Model file for the job. Use its own axes, mm. A direction names the side the tool comes from. Coordinates: 2 decimals unless noted, no trailing zeros. Order: outer loops, then holes, each group sorted by start corner. A loop starts at its lowest first (then second) coordinate and runs counter-clockwise, first axis right, second up. Notation, with made-up numbers: M 2,78.5 L 55,78.5 A30 ccw 55,105.5 Z; hole C 40.25,25.5 d3. An arc over 180 degrees is marked long. Return JSON: item names as keys, results as strings.
```python
from build123d import *

# Parameters (mm, degrees)
F0_R     = 24.5
F1_DEPTH = 17
F2_T     = 2
F3_W     = 1
F3_H     = 12
F4_DEPTH = 3


with BuildPart() as f1:
    # F0 (on Top) → F1 (new body)
    with BuildSketch(Plane.XY):
        Circle(F0_R)
    extrude(amount=F1_DEPTH)

    # F2
    f2_openings = [f1.faces().sort_by_distance(p)[0] for p in [
        (0, 0, 17),
    ]]
    offset(amount=F2_T, openings=f2_openings, kind=Kind.INTERSECTION)

    # F3 (on face) → F4 (join)
    with BuildSketch(Plane.XY):
        with Locations((-16.7093845084, 0.0996340905)):
            Rectangle(F3_W, F3_H)
        Polygon((3.322254178, -17.9535812131), (13.7145590234, -11.9535812131), (13.2145590234, -11.0875558093), (2.822254178, -17.0875558093), align=None)
        Polygon((13.8871303304, 11.8539471225), (3.494825485, 17.8539471225), (2.994825485, 16.9879217187), (13.3871303304, 10.9879217187), align=None)
    extrude(amount=F4_DEPTH)


solid = f1.part
```
Item 1: Saw through at C-C (z = 6.25). Write the cut outline in (x, y).
Check result:
{"outline": "C 0,0 d53; hole C 0,0 d49"}
Item 2: Pull direction X, two halves, no side cores. Call faces 3 (the cylindrical face through (14.246, 22.345, 7.367)), 4 (the flat face through (8.12, 14.03, 1.48)), 5 (the flat face through (7.73, -23.43, 17)): +X half, -X half, draft (parallel to the pull), parting line (faces both ways), or undercut.
Check result:
{"face 3": "parting line", "face 4": "undercut", "face 5": "draft"}
Item 3: Saw through at B-B (x = 0). Write the cut outline in (y, z).
Check result:
{"outline": "M -26.5,-2 L 26.5,-2 L 26.5,17 L 24.5,17 L 24.5,0 L -24.5,0 L -24.5,17 L -26.5,17 Z"}
Item 4: 3-axis set-ups, long thin cutter, end or side, ignore diameter. For faces 1 (the flat face through (0, 0, -2)), 2 (the flat face through (8.091, -14.046, 1.479)): which of +Z, -Z, +X, -X, +Y, -Y reach the whole face in a straight line?
Check result:
{"face 1": "-Z, +X, -X, +Y, -Y", "face 2": "+Z"}
Item 5: Saw through at A-A (y = 0). Write the cut outline in (x, z).
Check result:
{"outline": "M -26.5,-2 L 26.5,-2 L 26.5,17 L 24.5,17 L 24.5,0 L -16.21,0 L -16.21,3 L -17.21,3 L -17.21,0 L -24.5,0 L -24.5,17 L -26.5,17 Z"}
Item 6: Saw through at D-D (x = -21.5). Write the cut outline in (y, z).
Check result:
{"outline": "M -15.49,-2 L 15.49,-2 L 15.49,17 L 11.75,17 L 11.75,0 L -11.75,0 L -11.75,17 L -15.49,17 Z"}
Item 7: Wall check: line 1 (Y direction, x = 0, z = 9.75); line 2 (Y direction, x = 4, z = 1); line 3 (Z direction, x = -15, y = 3.5). Give the ranges that are in metal, low to high.
Check result:
{"line 1": "y = -26.5 to -24.5, 24.5 to 26.5", "line 2": "y = -26.2 to -24.17, -17.56 to -16.41, 16.41 to 17.56, 24.17 to 26.2", "line 3": "z = -2 to 0"}
Item 8: Drop flat-ended pins along their axis: pin 1 Ø7.5 at (x, y) = (6.5, 13.5) entering from +Z; pin 2 Ø8 at (y, z) = (-14.5, 6) entering from +X; pin 3 Ø5 at (y, z) = (9, 13.5) entering from +X. Give the stop position or say it passes through.
Check result:
{"pin 1": "stops at z = 3", "pin 2": "stops at x = 24.33", "pin 3": "stops at x = 25.69"}
